Can you work these out from the model? Positions are in its coordinate system, mm. Face numbers are marked on the shaded views. A direction names the side the tool comes from. Coordinates: 2 decimals unless noted, no trailing zeros. Loops run counter-clockwise (first coordinate to the right, second up) from the corner with the lowest first, then second, coordinate; pieces in that order, holes last. Notation, with made-up numbers: M 16,53 L 23,53 A29 ccw 23,83 Z; hole C 65.5,5.5 d1. An arc over 180 degrees is marked long. Answer as a JSON object with one key per item and string values. Group by question number.
Item 1: Suppose I cut it at D-D (z = 2.5). Count the separate pieces of the cut face and the enclosed holes in it, then the cut area to 3 significant figures.
Item 2: Suppose I cut it at C-C (y = 19.25). Write out the boundary of the cut face in (x, z).
Item 3: We'd pull the mould along Y, two halves only. Please class the marked faces 4, 5 and 6: +Y half, -Y half, draft (parallel to the pull), parting line (faces both ways), or undercut.
Item 4: I'm going to push flat-ended pins straight in: pin 1 Ø1.5 at (x, z) = (-12.5, 10.5) entering from +Y; pin 2 Ø4 at (y, z) = (-31, 2) entering from -X; pin 3 Ø1 at (y, z) = (-29, 7.5) entering from +X; pin 4 Ø4 at (x, y) = (-33.34, -19.25) entering from -Z. Where does each tip first touch, or does it pass through?
Item 5: If I drill on line 1 (Y direction, x = 0, z = 2.5); line 2 (Y direction, x = 0, z = 10.4); line 3 (Y direction, x = 31, z = 5.5), over which ranges is the centre line in solid material (lowest first)?
Item 6: Suppose I cut it at B-B (x = 24.5). Write out the boundary of the cut face in (y, z) (3 decimals), then the cut area to 3 significant figures.
Item 7: Which directions (+Z, -Z, +X, -X, +Y, -Y) give clear straight access to the entire face, cutting with the end or side of a thin tool? Please do the marked faces 1, 2 and 3.
Item 8: Suppose I cut it at A-A (x = -29). Write out the boundary of the cut face in (y, z), then the cut area to 3 significant figures.
```python
from build123d import *

# Parameters (mm, degrees)
SKETCH_1_R      = 46
SKETCH_1_R_2    = 34.3
SKETCH_1_R_3    = 1.6
EXTRUDE_1_DEPTH = 12
EXTRUDE_START   = -2.3
SKETCH_4_R      = 34.3
SKETCH_4_R_2    = 27.488330285
EXTRUDE_2_DEPTH = 2.3


with BuildPart() as part:
    # 草图1 → 凸台-拉伸1 (new body)
    with BuildSketch(Plane.XY):
        Circle(SKETCH_1_R)
        Circle(SKETCH_1_R_2, mode=Mode.SUBTRACT)
        with Locations((0, 38.5)):
            Circle(SKETCH_1_R_3, mode=Mode.SUBTRACT)
        with Locations((33.341978046, 19.25)):
            Circle(SKETCH_1_R_3, mode=Mode.SUBTRACT)
        with Locations((33.341978046, -19.25)):
            Circle(SKETCH_1_R_3, mode=Mode.SUBTRACT)
        with Locations((0, -38.5)):
            Circle(SKETCH_1_R_3, mode=Mode.SUBTRACT)
        with Locations((-33.341978046, -19.25)):
            Circle(SKETCH_1_R_3, mode=Mode.SUBTRACT)
        with Locations((-33.341978046, 19.25)):
            Circle(SKETCH_1_R_3, mode=Mode.SUBTRACT)
        with BuildLine():
            ThreePointArc((-7.974877173, 40.216928452), (-19.999395147, 35.791398321), (-30.070678328, 27.87031225))
            ThreePointArc((-30.070678328, 27.87031225), (-29.936509665, 24.337325019), (-26.403522434, 24.471493683))
            ThreePointArc((-26.403522434, 24.471493683), (-17.56044452, 31.426593647), (-7.002331176, 35.312424982))
            ThreePointArc((-7.002331176, 35.312424982), (-5.03635244, 38.250949715), (-7.974877173, 40.216928452))
        make_face(mode=Mode.SUBTRACT)
        with BuildLine():
            ThreePointArc((30.841443115, 27.01491045), (20.996562609, 35.215683418), (9.101059256, 39.977127466))
            ThreePointArc((9.101059256, 39.977127466), (6.108486895, 38.09444038), (7.991173981, 35.101868019))
            ThreePointArc((7.991173981, 35.101868019), (18.436006193, 30.921087879), (27.080291515, 23.720409175))
            ThreePointArc((27.080291515, 23.720409175), (30.608117952, 23.487084013), (30.841443115, 27.01491045))
        make_face(mode=Mode.SUBTRACT)
        with BuildLine():
            ThreePointArc((38.816320288, -13.202018002), (40.995957756, -0.575714903), (39.171737584, 12.106815216))
            ThreePointArc((39.171737584, 12.106815216), (36.044996559, 13.757115361), (34.394696415, 10.630374336))
            ThreePointArc((34.394696415, 10.630374336), (35.996450713, -0.505505768), (34.082622692, -11.592015806))
            ThreePointArc((34.082622692, -11.592015806), (35.644470392, -14.763865702), (38.816320288, -13.202018002))
        make_face(mode=Mode.SUBTRACT)
        with BuildLine():
            ThreePointArc((7.974877173, -40.216928452), (19.999395147, -35.791398321), (30.070678328, -27.87031225))
            ThreePointArc((30.070678328, -27.87031225), (29.936509665, -24.337325019), (26.403522434, -24.471493683))
            ThreePointArc((26.403522434, -24.471493683), (17.56044452, -31.426593647), (7.002331176, -35.312424982))
            ThreePointArc((7.002331176, -35.312424982), (5.03635244, -38.250949715), (7.974877173, -40.216928452))
        make_face(mode=Mode.SUBTRACT)
        with BuildLine():
            ThreePointArc((-30.841443115, -27.01491045), (-20.996562609, -35.215683418), (-9.101059256, -39.977127466))
            ThreePointArc((-9.101059256, -39.977127466), (-6.108486895, -38.09444038), (-7.991173981, -35.101868019))
            ThreePointArc((-7.991173981, -35.101868019), (-18.436006193, -30.921087879), (-27.080291515, -23.720409175))
            ThreePointArc((-27.080291515, -23.720409175), (-30.608117952, -23.487084013), (-30.841443115, -27.01491045))
        make_face(mode=Mode.SUBTRACT)
        with BuildLine():
            ThreePointArc((-38.816320288, 13.202018002), (-40.995957756, 0.575714903), (-39.171737584, -12.106815216))
            ThreePointArc((-39.171737584, -12.106815216), (-36.044996559, -13.757115361), (-34.394696415, -10.630374336))
            ThreePointArc((-34.394696415, -10.630374336), (-35.996450713, 0.505505768), (-34.082622692, 11.592015806))
            ThreePointArc((-34.082622692, 11.592015806), (-35.644470392, 14.763865702), (-38.816320288, 13.202018002))
        make_face(mode=Mode.SUBTRACT)
    extrude(amount=EXTRUDE_1_DEPTH)

    # 草图4 → 凸台-拉伸2 (add)
    with BuildSketch(Plane.XY.offset(12).offset(EXTRUDE_START)):
        Circle(SKETCH_4_R)
        Circle(SKETCH_4_R_2, mode=Mode.SUBTRACT)
    extrude(amount=EXTRUDE_2_DEPTH)


solid = part.part
```
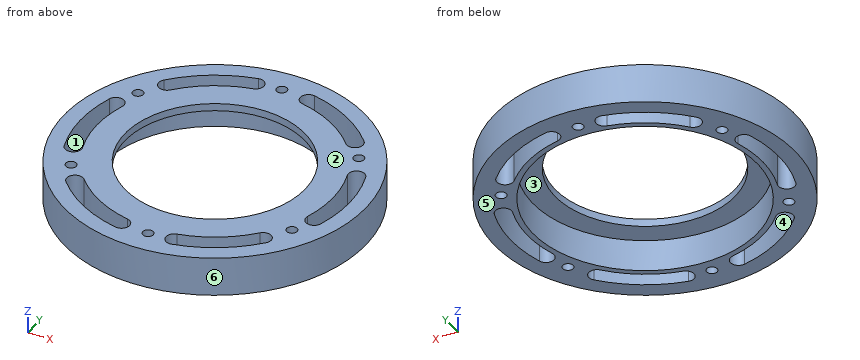
From the geometry:
{
 "1": {"separate pieces": "1", "enclosed holes": "13", "area": "2,060 mm2"},
 "2": {"outline": "M -41.78,0 L -34.94,0 L -34.94,12 L -41.78,12 Z; M -31.74,0 L -28.39,0 L -28.39,9.7 L -19.62,9.7 L -19.62,12 L -31.74,12 Z; M 19.62,9.7 L 28.39,9.7 L 28.39,0 L 31.74,0 L 31.74,12 L 19.62,12 Z; M 34.94,0 L 41.78,0 L 41.78,12 L 34.94,12 Z"},
 "3": {"face 4": "undercut", "face 5": "draft", "face 6": "parting line"},
 "4": {"pin 1": "y = 44.47", "pin 2": "x = -35.71", "pin 3": "x = 36.11", "pin 4": "z = 0"},
 "5": {"line 1": "-46 to -40.1, -36.9 to -34.3, 34.3 to 36.9, 40.1 to 46", "line 2": "-46 to -40.1, -36.9 to -27.49, 27.49 to 36.9, 40.1 to 46", "line 3": "-33.99 to -14.68, 14.68 to 23.92, 26.81 to 33.99"},
 "6": {"outline": "M -38.933,0 L -32.875,0 L -32.875,12 L -38.933,12 Z; M -26.377,0 L -24.005,0 L -24.005,9.7 L -12.464,9.7 L -12.464,12 L -26.377,12 Z; M 12.464,9.7 L 24.005,9.7 L 24.005,0 L 26.377,0 L 26.377,12 L 12.464,12 Z; M 32.875,0 L 38.933,0 L 38.933,12 L 32.875,12 Z", "area": "255 mm2"},
 "7": {"face 1": "+Z, -Z", "face 2": "+Z, +X, -X, +Y, -Y", "face 3": "-Z"},
 "8": {"outline": "M -35.71,0 L -28.98,0 L -28.98,12 L -35.71,12 Z; M -22.87,0 L -18.32,0 L -18.32,9.7 L 18.32,9.7 L 18.32,0 L 23.79,0 L 23.79,12 L -22.87,12 Z; M 28.98,0 L 35.71,0 L 35.71,12 L 28.98,12 Z", "area": "366 mm2"}
}
